```python
from build123d import *

# Parameters (mm, degrees)
BOSS_EXTRUDE1_DEPTH     = 17.526
CUT_EXTRUDE1_DEPTH      = 69.450165313
CUT_EXTRUDE1_DEPTH_BACK = 69.450165313
SKETCH2_W               = 8.819814413
SKETCH2_H               = 7.366
SKETCH2_W_2             = 48.073484567
SKETCH2_W_3             = 56.89329898


with BuildPart() as part:
    # Sketch1 → Boss-Extrude1 (new body)
    with BuildSketch(Plane.XY):
        Polygon((10, -10), (15, -10), (63.073484567, -10), (63.073484567, -5), (15, -5), (15, 15), (-15, 15), (-15, -5), (-63.073484567, -5), (-63.073484567, -10), (-15, -10), (-10, -10), (-10, 10), (10, 10), align=None)
    extrude(amount=BOSS_EXTRUDE1_DEPTH)

    # Sketch2 → Cut-Extrude1 (cut, two sides: drawn at the far end of the back side and taken through both)
    with BuildSketch(Plane(origin=(0, -5, 0), x_dir=(1, 0, 0), z_dir=(0, 1, 0)).offset(-CUT_EXTRUDE1_DEPTH_BACK)):
        with Locations((-67.483391774, -8.763)):
            Rectangle(SKETCH2_W, SKETCH2_H)
        with Locations((-39.036742284, -8.763)):
            Rectangle(SKETCH2_W_2, SKETCH2_H)
        with Locations((43.44664949, -8.763)):
            Rectangle(SKETCH2_W_3, SKETCH2_H)
    extrude(amount=CUT_EXTRUDE1_DEPTH + CUT_EXTRUDE1_DEPTH_BACK, mode=Mode.SUBTRACT)


solid = part.part
```
Geometry: final body of the model. Coordinates: model frame, mm. A direction names the side the tool comes from. Round coordinates to 2 decimals unless told otherwise and drop trailing zeros. Order: outer loops, then holes, each group sorted by start corner. A loop starts at its lowest first (then second) coordinate and runs counter-clockwise, first axis right, second up. Notation, with made-up numbers: M -35.75,-11 L -22.75,-11 A13 ccw -22.75,-1 Z; hole C 54.25,34 d1. An arc over 180 degrees is marked long. Use one line per item in the form item = value. Start each with the question number.
Q1. Cut plane C-C (z = 13.5). Return loops of the section in (x, y), and give its area (3 significant figures).
Q2. Cut plane D-D (y = 13.75). Return loops of the section in (x, z), and give its area (3 significant figures).
Q3. Cut plane B-B (x = 52). Return loops of the section in (y, z).
Q4. Pin query (flat end, axial travel): pin 1 Ø1.5 at (x, z) = (43, 14) entering from +Y; pin 2 Ø1.5 at (x, z) = (-23.5, 11.5) entering from +Y; pin 3 Ø5 at (y, z) = (4.5, 9) entering from +X; pin 4 Ø9 at (y, z) = (3.5, 12.5) entering from -X. Return the tip coordinate at first contact, or that it passes through.
Q5. Mould query, pull axis Z, two halves, no side actions, for faces 1 (the face through (39, -8, 5.08)), 2 (the face through (-1, 11, 17.526)), 3 (the face through (36, -10, 13)). Classes: +Z half, -Z half, draft (parallel to the pull), parting line (faces both ways), or undercut.
Q6. Material intervals for line 1 (X direction, y = 8.25, z = 14.5); line 2 (X direction, y = -8, z = 12.5); line 3 (Y direction, x = -47, z = 13), sorted ascending. Write a range as [from, to].
Q7. Access query for faces 4 (the face through (39, -8, 12.446)), 5 (the face through (39, -5, 15)), 6 (the face through (-39, -5, 15)), 7 (the face through (-10, 0, 9)). Directions: +Z, -Z, +X, -X, +Y, -Y. A direction counts if a zero-diameter tool reaches every point of the face in a straight line with its end or side. Return the directions, or none.
Q8. Cut plane A-A (y = 7.5). Return loops of the section in (x, z), and give its area (3 significant figures).
Geometry results:
q1.outline = M -63.07,-10 L -10,-10 L -10,10 L 10,10 L 10,-10 L 63.07,-10 L 63.07,-5 L 15,-5 L 15,15 L -15,15 L -15,-5 L -63.07,-5 Z
q1.area = 831 mm^2
q2.outline = M -15,0 L 15,0 L 15,17.53 L -15,17.53 Z
q2.area = 526 mm^2
q3.outline = M -10,0 L -5,0 L -5,5.08 L -10,5.08 Z; M -10,12.45 L -5,12.45 L -5,17.53 L -10,17.53 Z
q4.pin_1 = -5
q4.pin_2 = through
q4.pin_3 = 15
q4.pin_4 = -15
q5.face_1 = undercut
q5.face_2 = +Z half
q5.face_3 = draft
q6.line_1 = [-15, -10], [10, 15]
q6.line_2 = [-63.07, -10], [10, 63.07]
q6.line_3 = [-10, -5]
q7.face_4 = +X, +Y, -Y
q7.face_5 = +Z, -Z, +X, +Y
q7.face_6 = +Z, -Z, -X, +Y
q7.face_7 = +Z, -Z, -Y
q8.outline = M -15,0 L -10,0 L -10,17.53 L -15,17.53 Z; M 10,0 L 15,0 L 15,17.53 L 10,17.53 Z
q8.area = 175 mm^2
